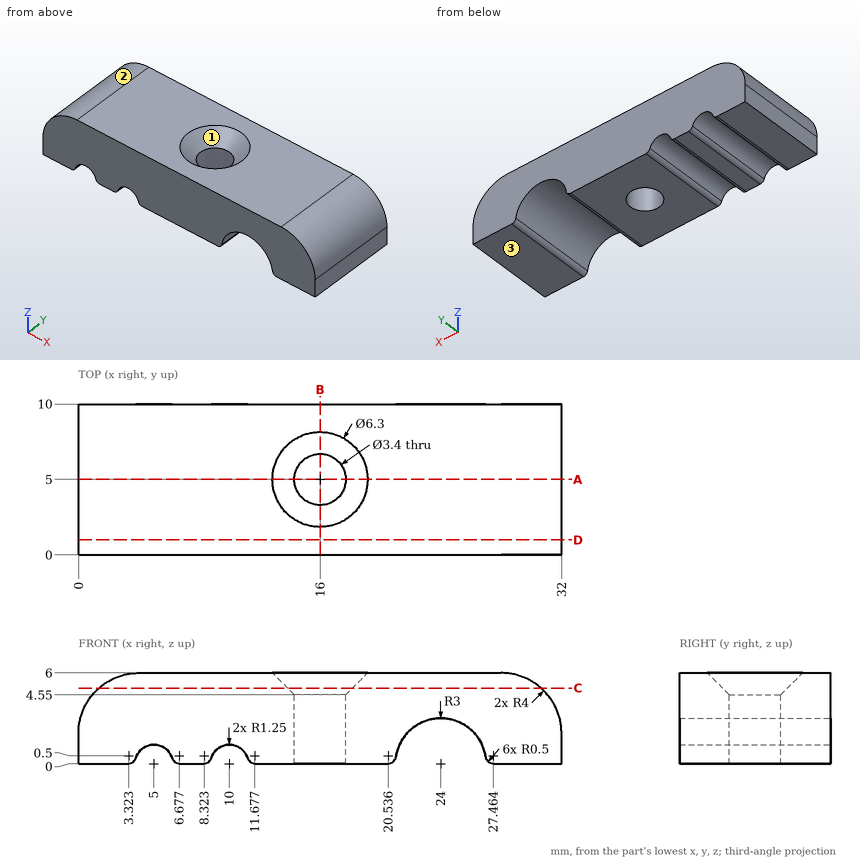
Can you work these out from the drawing? Everything is in mm from the part's minimum corner. Give positions to 0.01 mm unless a question says otherwise; leave off trailing zeros. Order: outer loops, then holes, each group sorted by start corner. A loop starts at its lowest first (then second) coordinate and runs counter-clockwise, first axis right, second up. Notation, with made-up numbers: M 61.25,15 L 70.25,15 A25 ccw 70.25,48 Z; hole C 10.5,23 d3. An arc over 180 degrees is marked long. Use a Markdown table: item, result. Add a question column.
1. I need wall thicknesses on probe 1 along Y at (x, z) = (16, 2.9); probe 2 along X at (y, z) = (5, 1.5); probe 3 along X at (y, z) = (5, 2.25). Which ranges of each line are inside material? Lowest first, please. Write a range as from..to.
2. Suppose I cut it at C-C (z = 5). List the corners of the cut face in (x, y) for me.
3. Suppose I cut it at A-A (y = 5). List the corners of the cut face in (x, z) for me.
4. Suppose I cut it at D-D (y = 1). List the corners of the cut face in (x, z) for me, and give its area (3 significant figures).
5. For pin 1 Ø2 at (x, y) = (3.5, 7) entering from -Z; pin 2 Ø4 at (x, y) = (16, 5) entering from +Z; pin 3 Ø2 at (y, z) = (3, 3.5) entering from -X, each with a flat end and sliding along its axis, tell me the tip position at first contact or that it passes through.
6. Suppose I cut it at B-B (x = 16). List the corners of the cut face in (y, z) for me.
7. If we mould it in two halves opening along X, with no side actions, what happens to the marked faces 1, 2 and 3? For each: +X half, -X half, draft (parallel to the pull), parting line (faces both ways), or undercut.
Results list:
| question | item | result |
|---|---|---|
| 1 | probe 1 | y = 0..3.3, 6.7..10 |
| 1 | probe 2 | x = 0..14.3, 17.7..21.4, 26.6..32 |
| 1 | probe 3 | x = 0.01..14.3, 17.7..22.02, 25.98..31.99 |
| 2 | outline | M 1.35,0 L 30.65,0 L 30.65,10 L 1.35,10 Z; hole C 16,5 d4.3 |
| 3 | outline | M 0,0 L 3.32,0 A0.5 ccw 3.8,0.36 A1.25 cw 6.2,0.36 A0.5 ccw 6.68,0 L 8.32,0 A0.5 ccw 8.8,0.36 A1.25 cw 11.2,0.36 A0.5 ccw 11.68,0 L 14.3,0 L 14.3,4.55 L 12.85,6 L 4,6 A4 ccw 0,2 Z; M 17.7,0 L 20.54,0 A0.5 ccw 21.03,0.43 A3 cw 26.97,0.43 A0.5 ccw 27.46,0 L 32,0 L 32,2 A4 ccw 28,6 L 19.15,6 L 17.7,4.55 Z |
| 4 | outline | M 0,0 L 3.32,0 A0.5 ccw 3.8,0.36 A1.25 cw 6.2,0.36 A0.5 ccw 6.68,0 L 8.32,0 A0.5 ccw 8.8,0.36 A1.25 cw 11.2,0.36 A0.5 ccw 11.68,0 L 20.54,0 A0.5 ccw 21.03,0.43 A3 cw 26.97,0.43 A0.5 ccw 27.46,0 L 32,0 L 32,2 A4 ccw 28,6 L 4,6 A4 ccw 0,2 Z |
| 4 | area | 166 mm² |
| 5 | pin 1 | stops at z = 0 |
| 5 | pin 2 | stops at z = 4.85 |
| 5 | pin 3 | stops at x = 0.03 |
| 6 | outline | M 0,0 L 3.3,0 L 3.3,4.55 L 1.85,6 L 0,6 Z; M 6.7,0 L 10,0 L 10,6 L 8.15,6 L 6.7,4.55 Z |
| 7 | face 1 | undercut |
| 7 | face 2 | -X half |
| 7 | face 3 | draft |
